Geometry check sheet. Reference: the model listing, model coordinates, mm. A direction names the side the tool comes from. Coordinates: 2 decimals unless noted, no trailing zeros. Loops run counter-clockwise (first coordinate to the right, second up) from the corner with the lowest first, then second, coordinate; pieces in that order, holes last.
from build123d import *

# Parameters (mm, degrees)
F0_W      = 124.8
F0_H      = 81
F1_DEPTH  = 63
F2_W      = 123.1
F2_H      = 79.3
F3_DEPTH  = 3
F4_W      = 123.1
F4_H      = 79.3
F5_DEPTH  = 3
F6_W      = 120.8
F6_H      = 77
F7_DEPTH  = 60.001
F8_W      = 12
F8_H      = 10
F9_DEPTH  = 81
F10_W     = 12
F10_H     = 10
F11_DEPTH = 81
F12_W     = 12
F12_H     = 10
F13_DEPTH = 124.8
F14_R     = 1.5
F15_DEPTH = 50.001
F16_R     = 1.5
F17_DEPTH = 50.001
F18_R     = 1.5
F19_DEPTH = 50.001
F20_R     = 1.5
F21_DEPTH = 50.001
F22_R     = 1.5
F23_DEPTH = 50.001
F24_W     = 10
F24_H     = 10
F25_DEPTH = 81
F26_R     = 1.5
F27_DEPTH = 50.001
F28_W     = 10
F28_H     = 10
F29_DEPTH = 69
F30_R     = 1.5
F31_DEPTH = 50.001
F32_W     = 25
F32_H     = 25
F33_DEPTH = 25
F34_R     = 1.5
F35_DEPTH = 50.001


with BuildPart() as f1:
    # F0 (on Top) → F1 (new body)
    with BuildSketch(Plane.XY):
        Rectangle(F0_W, F0_H)
    extrude(amount=F1_DEPTH)

    # F2 (on face) → F3 (cut)
    with BuildSketch(Plane.XY.offset(63)):
        Rectangle(F2_W, F2_H)
    extrude(amount=-F3_DEPTH, mode=Mode.SUBTRACT)

    # F4 (on face) → F5 (cut)
    with BuildSketch(Plane(origin=(0, 0, 0), x_dir=(1, 0, 0), z_dir=(0, 0, -1))):
        Rectangle(F4_W, F4_H)
    extrude(amount=-F5_DEPTH, mode=Mode.SUBTRACT)

    # F6 (on face) → F7 (cut, through all)
    with BuildSketch(Plane.XY.offset(60)):
        Rectangle(F6_W, F6_H)
    extrude(amount=-F7_DEPTH, mode=Mode.SUBTRACT)

    # F8 (on face) → F9 (join)
    with BuildSketch(Plane.XZ.offset(40.5)):
        with Locations((-56.4, 45)):
            Rectangle(F8_W, F8_H)
    extrude(amount=-F9_DEPTH)

    # F10 (on face) → F11 (join)
    with BuildSketch(Plane.XZ.offset(40.5)):
        with Locations((56.4, 45)):
            Rectangle(F10_W, F10_H)
    extrude(amount=-F11_DEPTH)

    # F12 (on face) → F13 (join)
    with BuildSketch(Plane(origin=(-62.4, 0, 0), x_dir=(0, -1, 0), z_dir=(-1, 0, 0))):
        with Locations((-34.5, 45)):
            Rectangle(F12_W, F12_H)
    extrude(amount=-F13_DEPTH)

    # F14 (on face) → F15 (cut, through all)
    with BuildSketch(Plane.XY.offset(50)):
        with Locations((-55.4, 33.5)):
            Circle(F14_R)
    extrude(amount=-F15_DEPTH, mode=Mode.SUBTRACT)

    # F16 (on face) → F17 (cut, through all)
    with BuildSketch(Plane.XY.offset(50)):
        with Locations((55.4, 33.5)):
            Circle(F16_R)
    extrude(amount=-F17_DEPTH, mode=Mode.SUBTRACT)

    # F18 (on face) → F19 (cut, through all)
    with BuildSketch(Plane.XY.offset(50)):
        with Locations((-55.4, -22.5)):
            Circle(F18_R)
    extrude(amount=-F19_DEPTH, mode=Mode.SUBTRACT)

    # F20 (on face) → F21 (cut, through all)
    with BuildSketch(Plane.XY.offset(50)):
        with Locations((-8.1, 33.5)):
            Circle(F20_R)
    extrude(amount=-F21_DEPTH, mode=Mode.SUBTRACT)

    # F22 (on face) → F23 (cut, through all)
    with BuildSketch(Plane.XY.offset(50)):
        with Locations((10.06, 33.5)):
            Circle(F22_R)
    extrude(amount=-F23_DEPTH, mode=Mode.SUBTRACT)

    # F24 (on face) → F25 (join)
    with BuildSketch(Plane.XZ.offset(40.5)):
        with Locations((31, 45)):
            Rectangle(F24_W, F24_H)
    extrude(amount=-F25_DEPTH)

    # F26 (on face) → F27 (cut, through all)
    with BuildSketch(Plane.XY.offset(50)):
        with Locations((31, -22.5)):
            Circle(F26_R)
    extrude(amount=-F27_DEPTH, mode=Mode.SUBTRACT)

    # F28 (on face) → F29 (join)
    with BuildSketch(Plane.XZ.offset(40.5)):
        with Locations((-8.1, 45)):
            Rectangle(F28_W, F28_H)
    extrude(amount=-F29_DEPTH)

    # F30 (on face) → F31 (cut, through all)
    with BuildSketch(Plane.XY.offset(50)):
        with Locations((-8.1, -14.5)):
            Circle(F30_R)
    extrude(amount=-F31_DEPTH, mode=Mode.SUBTRACT)

    # F32 (on face) → F33 (cut)
    with BuildSketch(Plane(origin=(0, 40.5, 0), x_dir=(-1, 0, 0), z_dir=(0, 1, 0))):
        with Locations((26.9, 27.5)):
            Rectangle(F32_W, F32_H)
    extrude(amount=-F33_DEPTH, mode=Mode.SUBTRACT)

    # F34 (on face) → F35 (cut, through all)
    with BuildSketch(Plane.XY.offset(50)):
        with Locations((55.4, -24.54)):
            Circle(F34_R)
    extrude(amount=-F35_DEPTH, mode=Mode.SUBTRACT)


solid = f1.part
(1) Access from +Z, -Z, +X, -X, +Y, -Y to the whole of each face (thin tool, end or side, straight path). Record for faces 1 (the flat face through (61.55, 1, 1)), 2 (the flat face through (36, -5, 45)), 3 (the flat face through (-60.4, -1, 55)).
Findings:
face 1: -Z
face 2: +Z, -Z
face 3: +Z
(2) Sectioned sample at D-D on z = 4.5. Record the cut outline in (x, y), and give its area (3 significant figures).
Findings:
outline: (-62.4, -40.5) - (62.4, -40.5) - (62.4, 40.5) - (-62.4, 40.5) - close; hole (-60.4, -38.5) - (60.4, -38.5) - (60.4, 38.5) - (-60.4, 38.5) - close
area: 807 mm2
(3) Sectioned sample at B-B on y = 14.5. State how many separate pieces and enclosed holes the cut face has, and give its area (3 significant figures).
Findings:
separate pieces: 4
enclosed holes: 0
area: 638 mm2
(4) Gauge pin test, flat end, axial feed: pin 1 Ø4 at (x, y) = (-55.4, -22.5) entering from +Z. Record the tip position at first contact, or that the pin passes through.
Findings:
pin 1: stops at z = 50
(5) Sectioned sample at A-A on x = 31. Record the cut outline in (y, z).
Findings:
outline: (-40.5, 0) - (-39.65, 0) - (-39.65, 3) - (-38.5, 3) - (-38.5, 40) - (-24, 40) - (-24, 50) - (-38.5, 50) - (-38.5, 60) - (-39.65, 60) - (-39.65, 63) - (-40.5, 63) - close; (-21, 40) - (38.5, 40) - (38.5, 3) - (39.65, 3) - (39.65, 0) - (40.5, 0) - (40.5, 63) - (39.65, 63) - (39.65, 60) - (38.5, 60) - (38.5, 50) - (-21, 50) - close
(6) Draft check along X on faces 4 (the cylindrical face through (-56.51, -21.49, 45.07)), 5 (the flat face through (-1, -40.5, 32)). Enter one of: +X half, -X half, draft (parallel to the pull), parting line (faces both ways), or undercut.
Findings:
face 4: undercut
face 5: draft
(7) Scan lines: L1, parallel to Y at x = -8.1, z = 42.5; L2, parallel to X at y = 1.5, z = 44; L3, parallel to X at y = 12, z = 59. Record each from-to range of solid material in increasing order.
Findings:
L1: y = -40.5 to -16, -13 to 32, 35 to 40.5
L2: x = -62.4 to -50.4, -13.1 to -3.1, 26 to 36, 50.4 to 62.4
L3: x = -62.4 to -60.4, 60.4 to 62.4
(8) Sectioned sample at C-C on x = 10.06. Record the cut outline in (y, z).
Findings:
outline: (-40.5, 0) - (-39.65, 0) - (-39.65, 3) - (-38.5, 3) - (-38.5, 60) - (-39.65, 60) - (-39.65, 63) - (-40.5, 63) - close; (28.5, 40) - (32, 40) - (32, 50) - (28.5, 50) - close; (35, 40) - (38.5, 40) - (38.5, 3) - (39.65, 3) - (39.65, 0) - (40.5, 0) - (40.5, 63) - (39.65, 63) - (39.65, 60) - (38.5, 60) - (38.5, 50) - (35, 50) - close
